Here's how the part is built. I have some questions about the finished solid (model axes, mm). Face numbers are marked on the shaded views. A direction names the side the tool comes from. Coordinates: 2 decimals unless noted, no trailing zeros. Order: outer loops, then holes, each group sorted by start corner. A loop starts at its lowest first (then second) coordinate and runs counter-clockwise, first axis right, second up. Notation, with made-up numbers: (17.25, 39) - (66.25, 39) arc R9 ccw to (66.25, 49) - close; hole circle Ø9 at (2, -37.5). An arc over 180 degrees is marked (long way). Answer in a Markdown table with one row per item. Add a question column.
Item 1: If I drill on line 1 along Y through (x, z) = (-5.5, -11); line 2 along Z through (x, y) = (17.5, 7); line 3 along Y through (x, z) = (-6, 0), over which ranges is the centre line in solid material (lowest first)? Write a range as from..to.
Item 2: On a 3-axis mill with a long thin cutter (end or side, diameter ignored), from which of +Z, -Z, +X, -X, +Y, -Y can I reach the whole of each face in a straight line? I mean the marked faces 4, 5 and 6. Say none if no direction works.
Item 3: Thinking about a two-plate mould opening in Z: for the marked faces 1, 2 and 3, which applies, +Z half, -Z half, draft (parallel to the pull), parting line (faces both ways), or undercut?
Item 4: Will these pins go through, and if not, where does the flat tip stop? pin 1 Ø7.5 at (y, z) = (0, 0) entering from -X; pin 2 Ø2 at (x, y) = (-11.5, -53) entering from +Z; pin 3 Ø3 at (y, z) = (22, -57.5) entering from -X; pin 4 Ø10 at (x, z) = (8.5, -15.5) entering from -Y.
Item 5: I want a section at A-A (y = 0). Count the separate pieces of the cut face and the enclosed holes in it, plus the area to 3 significant figures.
Item 6: I want a section at B-B (x = -9.5). Please give me the cut outline in (y, z).
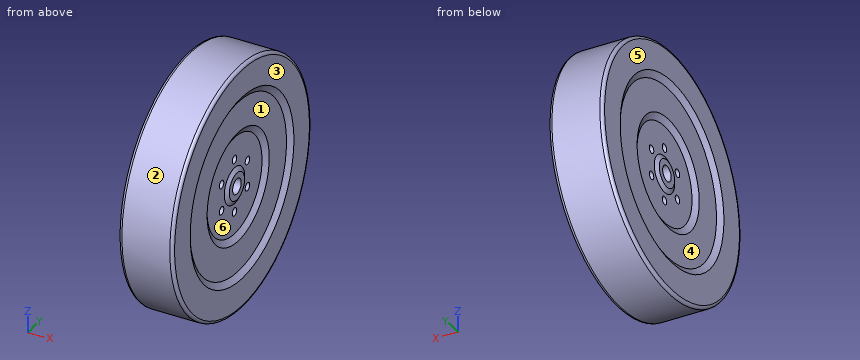
```python
from build123d import *

# Parameters (mm, degrees)
SKETCH3_R          = 3.3
CUT_EXTRUDE1_DEPTH = 39.259
FILLET1_R          = 2.54


with BuildPart() as part:
    # Sketch2 → Revolve1 (revolve)
    with BuildSketch(Plane(origin=(0, 0, 0), x_dir=(1, 0, 0), z_dir=(0, 1, 0))):
        Polygon((22.225, -101.6), (22.225, -76.2), (19.05, -71.063365236), (19.05, -45.663365236), (16.034, -40.4395), (16.034, -15.0395), (18.034, -11.2395), (18.034, -6.35), (-18.034, -6.35), (-18.034, -11.2395), (-16.034, -15.0395), (-16.034, -40.4395), (-19.05, -45.663365236), (-19.05, -71.063365236), (-22.225, -76.2), (-22.225, -101.6), align=None)
    revolve(axis=Axis((0, 0, 0), (1, 0, 0)))

    # Sketch3 → Cut-Extrude1 (cut, through all)
    with BuildSketch(Plane(origin=(16.034, 0, 0), x_dir=(0, 0, -1), z_dir=(1, 0, 0))):
        with Locations((22, 0)):
            Circle(SKETCH3_R)
        with Locations((11, -19.052558883)):
            Circle(SKETCH3_R)
        with Locations((-11, -19.052558883)):
            Circle(SKETCH3_R)
        with Locations((-22, 0)):
            Circle(SKETCH3_R)
        with Locations((-11, 19.052558883)):
            Circle(SKETCH3_R)
        with Locations((11, 19.052558883)):
            Circle(SKETCH3_R)
    extrude(amount=-CUT_EXTRUDE1_DEPTH, mode=Mode.SUBTRACT)

    # Fillet1
    fillet1_edges = [part.edges().sort_by_distance(p)[0] for p in [
        (22.225, 0, -101.6),
        (-22.225, 0, -101.6),
    ]]
    fillet(fillet1_edges, radius=FILLET1_R)


solid = part.part
```
Values follow:
| question | item | result |
|---|---|---|
| 1 | line 1 | y = -101..-22.35, -15.75..15.75, 22.35..101 |
| 1 | line 2 | z = -101.36..-42.4, -10.06..10.06, 42.4..101.36 |
| 1 | line 3 | y = -101.6..-6.35, 6.35..101.6 |
| 2 | face 4 | -X |
| 2 | face 5 | +Z, -Z, -X, +Y, -Y |
| 2 | face 6 | +X |
| 3 | face 1 | undercut |
| 3 | face 2 | parting line |
| 3 | face 3 | draft |
| 4 | pin 1 | passes through |
| 4 | pin 2 | stops at z = 87.28 |
| 4 | pin 3 | stops at x = -19.05 |
| 4 | pin 4 | stops at y = -101.06 |
| 5 | separate pieces | 4 |
| 5 | enclosed holes | 0 |
| 5 | area | 6,800 mm^2 |
| 6 | outline | circle Ø203.2 at (0, 0); hole circle Ø6.6 at (-19.05, -11); hole circle Ø6.6 at (-19.05, 11); hole circle Ø12.7 at (0, 0); hole circle Ø6.6 at (0, -22); hole circle Ø6.6 at (0, 22); hole circle Ø6.6 at (19.05, -11); hole circle Ø6.6 at (19.05, 11) |
